```python
from build123d import *

# Parameters (mm, degrees)
F0_R     = 39.6875
F0_R_2   = 2.38125
F1_DEPTH = 3.175


with BuildPart() as f1:
    # F0 (on Front) → F1 (new body)
    with BuildSketch(Plane.XZ):
        Circle(F0_R)
        with BuildLine():
            Line((-28.692183, -22.436528), (-11.631072, -10.022431))
            ThreePointArc((-11.631072, -10.022431), (-7.953459, -8.457568), (-3.961983, -8.661889))
            ThreePointArc((-3.961983, -8.661889), (-2.943387, -9.058813), (-1.886019, -9.33641))
            ThreePointArc((-1.886019, -9.33641), (1.46325, -11.517242), (3.518698, -14.944889))
            Line((3.518698, -14.944889), (10.024603, -35.016374))
            ThreePointArc((10.024603, -35.016374), (9.899166, -36.282225), (8.884648, -37.049602))
            ThreePointArc((8.884648, -37.049602), (-11.773547, -36.235253), (-28.965041, -24.751493))
            ThreePointArc((-28.965041, -24.751493), (-29.334751, -23.534353), (-28.692183, -22.436528))
        make_face(mode=Mode.SUBTRACT)
        with BuildLine():
            ThreePointArc((8.296642, -4.67882), (11.405717, -2.16739), (15.300772, -1.271745))
            Line((15.300772, -1.271745), (36.400324, -1.28669))
            ThreePointArc((36.400324, -1.28669), (37.565457, -1.797158), (37.981773, -2.999155))
            ThreePointArc((37.981773, -2.999155), (30.823547, -22.394618), (14.589379, -35.196023))
            ThreePointArc((14.589379, -35.196023), (13.317564, -35.171521), (12.472034, -34.221156))
            Line((12.472034, -34.221156), (5.937699, -14.158908))
            ThreePointArc((5.937699, -14.158908), (5.585871, -10.177722), (7.013626, -6.444741))
            ThreePointArc((7.013626, -6.444741), (7.705887, -5.598655), (8.296642, -4.67882))
        make_face(mode=Mode.SUBTRACT)
        with BuildLine():
            Line((-30.204778, 20.354619), (-13.126097, 7.964705))
            ThreePointArc((-13.126097, 7.964705), (-10.501379, 4.950657), (-9.462266, 1.091399))
            ThreePointArc((-9.462266, 1.091399), (-9.525, 0), (-9.462266, -1.091399))
            ThreePointArc((-9.462266, -1.091399), (-10.501379, -4.950657), (-13.126097, -7.964705))
            Line((-13.126097, -7.964705), (-30.204778, -20.354619))
            ThreePointArc((-30.204778, -20.354619), (-31.447436, -20.626491), (-32.490759, -19.898759))
            ThreePointArc((-32.490759, -19.898759), (-38.1, 0), (-32.490759, 19.898759))
            ThreePointArc((-32.490759, 19.898759), (-31.447436, 20.626491), (-30.204778, 20.354619))
        make_face(mode=Mode.SUBTRACT)
        with BuildLine():
            Line((10.024603, 35.016374), (3.518698, 14.944889))
            ThreePointArc((3.518698, 14.944889), (1.46325, 11.517242), (-1.886019, 9.33641))
            ThreePointArc((-1.886019, 9.33641), (-2.943387, 9.058813), (-3.961983, 8.661889))
            ThreePointArc((-3.961983, 8.661889), (-7.953459, 8.457568), (-11.631072, 10.022431))
            Line((-11.631072, 10.022431), (-28.692183, 22.436528))
            ThreePointArc((-28.692183, 22.436528), (-29.334751, 23.534353), (-28.965041, 24.751493))
            ThreePointArc((-28.965041, 24.751493), (-11.773547, 36.235253), (8.884648, 37.049602))
            ThreePointArc((8.884648, 37.049602), (9.899166, 36.282225), (10.024603, 35.016374))
        make_face(mode=Mode.SUBTRACT)
        Circle(F0_R_2, mode=Mode.SUBTRACT)
        with BuildLine():
            ThreePointArc((14.589379, 35.196023), (30.823547, 22.394618), (37.981773, 2.999155))
            ThreePointArc((37.981773, 2.999155), (37.565457, 1.797158), (36.400324, 1.28669))
            Line((36.400324, 1.28669), (15.300772, 1.271745))
            ThreePointArc((15.300772, 1.271745), (11.405717, 2.16739), (8.296642, 4.67882))
            ThreePointArc((8.296642, 4.67882), (7.705887, 5.598655), (7.013626, 6.444741))
            ThreePointArc((7.013626, 6.444741), (5.585871, 10.177722), (5.937699, 14.158908))
            Line((5.937699, 14.158908), (12.472034, 34.221156))
            ThreePointArc((12.472034, 34.221156), (13.317564, 35.171521), (14.589379, 35.196023))
        make_face(mode=Mode.SUBTRACT)
    extrude(amount=F1_DEPTH)


solid = f1.part
```
The listing builds one solid part. Answer for the finished solid, in the listing's coordinates (mm). Give positions to 0.01 mm unless a question says otherwise; leave off trailing zeros. Loops run counter-clockwise (first coordinate to the right, second up) from the corner with the lowest first, then second, coordinate; pieces in that order, holes last. Notation, with made-up numbers: M 18,21 L 65,21 A27 ccw 65,54 Z; hole C 38,-16.5 d11. An arc over 180 degrees is marked long. One line per item, written item: value.
1. Section A-A on z = 0 is taken. Determine the outline of the cut face in (x, y) (1 decimal).
Found:
outline: M -39.7,-3.2 L -38.1,-3.2 L -38.1,0 L -39.7,0 Z; M -9.5,-3.2 L -2.4,-3.2 L -2.4,0 L -9.5,0 Z; M 2.4,-3.2 L 39.7,-3.2 L 39.7,0 L 2.4,0 Z
2. Section D-D on z = 11 is taken. Determine the outline of the cut face in (x, y) (3 decimals).
Found:
outline: M -38.133,-3.175 L -36.478,-3.175 L -36.478,0 L -38.133,0 Z; M -17.31,-3.175 L -12.975,-3.175 L -12.975,0 L -17.31,0 Z; M 0.921,-3.175 L 5.51,-3.175 L 5.51,0 L 0.921,0 Z; M 36.478,-3.175 L 38.133,-3.175 L 38.133,0 L 36.478,0 Z
3. For a pull along Z with two mould halves and no side action, classify faces 1 (the face through (37.855, -1.565, 11.921)), 2 (the face through (5.58, -1.57, -10.23)), 3 (the face through (0, 0, 3)) as pulls with the +Z half, pulls with the -Z half, needs draft (parallel to the pull), parting line crosses it, or undercut.
Found:
face 1: parting line crosses it
face 2: undercut
face 3: needs draft
4. Section C-C on x = -24.5 is taken. Determine the outline of the cut face in (y, z) (3 decimals).
Found:
outline: M -3.175,-31.223 L 0,-31.223 L 0,-29.178 L -3.175,-29.178 Z; M -3.175,-19.386 L 0,-19.386 L 0,-16.216 L -3.175,-16.216 Z; M -3.175,16.216 L 0,16.216 L 0,19.386 L -3.175,19.386 Z; M -3.175,29.178 L 0,29.178 L 0,31.223 L -3.175,31.223 Z
5. Find the intervals of material crossed by probe 1 along Z at (x, y) = (-10.5, -0.1); probe 2 along Z at (x, y) = (0, -0.9); probe 3 along X at (y, z) = (-0.7, 18), in increasing order.
Found:
probe 1: -38.27 to -36.62, -9.32 to -4.95, 4.95 to 9.32, 36.62 to 38.27
probe 2: -39.69 to -38.1, -10.29 to -2.38, 2.38 to 10.29, 38.1 to 39.69
probe 3: -35.37 to -33.58, -26.96 to -22.59, 4.51 to 7.19, 33.58 to 35.37
6. Section B-B on x = 11.5 is taken. Determine the outline of the cut face in (y, z) (3 decimals), plus the area to 3 significant figures.
Found:
outline: M -3.175,-37.985 L 0,-37.985 L 0,-31.237 L -3.175,-31.237 Z; M -3.175,-2.122 L 0,-2.122 L 0,2.122 L -3.175,2.122 Z; M -3.175,31.237 L 0,31.237 L 0,37.985 L -3.175,37.985 Z
area: 56.3 mm^2
7. This flat-tipped pin is pushed along its axis until it touches: P1, Ø4, axis at x = 4, z = 5, coming from the +Y side. Where does it stop, or does it pass through?
Found:
P1: y = 0
